Read the model definition and answer for the solid it produces. Units are mm, in the model's axes. A direction names the side the tool comes from. Coordinates: 2 decimals unless noted, no trailing zeros. Loops run counter-clockwise (first coordinate to the right, second up) from the corner with the lowest first, then second, coordinate; pieces in that order, holes last. Notation, with made-up numbers: (35, 68) - (40, 68) arc R25 cw to (40, 91) - close; hole circle Ø4 at (84.25, 56.5). An arc over 180 degrees is marked (long way). Use one line per item in the form item = value. Start each with the question number.
1) A cutting plane is placed at A-A (z = 0). Give the vertices of the cut face in (x, y) (3 decimals), and give its area (3 significant figures).
2) A cutting plane is placed at D-D (y = -2). Give the vertices of the cut face in (x, z) (3 decimals).
3) Consider line 1 (Z direction, x = 0, y = -32.75); line 2 (X direction, y = -1.5, z = 4.5) (3 decimals); line 3 (Y direction, x = -5.75, z = -13.5) (3 decimals). Determine where each line is inside the solid, lowest interval first.
4) This flat-tipped pin is pushed along its axis until it touches: P1, Ø5, axis at x = 0, z = 0, coming from the -Y side. Where does it stop, or does it pass through?
5) The mould has two halves that part along X. Classify faces 1 (the face through (0, -12.725, 5)), 2 (the face through (12.7, -9, 0)), 3 (the face through (-12.7, -9, 0)), 4 (the face through (9, 19.05, 0)): released by +X, released by -X, zero draft, split by the parting line, or undercut.
6) A cutting plane is placed at C-C (y = -16). Give the vertices of the cut face in (x, z), and give its area (3 significant figures).
7) Which of the six approach directions +Z, -Z, +X, -X, +Y, -Y give full straight-line access (tool end or side, diameter ignored) to faces 5 (the face through (6.375, 3, 0)), 6 (the face through (2.539, -25.247, -1.947))?
8) A cutting plane is placed at B-B (x = 0). Give the vertices of the cut face in (y, z) (3 decimals).
from build123d import *

# Parameters (mm, degrees)
F0_W      = 25.4
F0_H      = 38.1
F1_DEPTH  = 19.05
F2_T      = -6.325
F1_FACE_W = 25.4
F1_FACE_H = 38.1
F3_DEPTH  = 19.075
F5_D      = 6.4
F5_DEPTH  = 50


with BuildPart() as f1:
    # F0 (on Top) → F1 (new body, symmetric)
    with BuildSketch(Plane.XY):
        Rectangle(F0_W, F0_H)
    extrude(amount=F1_DEPTH, both=True)

    # F2
    f2_openings = [f1.faces().sort_by_distance(p)[0] for p in [
        (0, 19.05, 0),
        (0, 0, 19.05),
        (0, 0, -19.05),
    ]]
    offset(amount=F2_T, openings=f2_openings)

    # F1_face (on face) → F3 (join)
    with BuildSketch(Plane.XZ.offset(19.05)):
        Rectangle(F1_FACE_W, F1_FACE_H)
    extrude(amount=F3_DEPTH)

    # F5
    with Locations(Plane.XZ.offset(38.125)):
        with Locations((0, 0)):
            Hole(F5_D / 2, depth=F5_DEPTH)


solid = f1.part
Found:
q1.outline = (-12.7, -38.125) - (-3.2, -38.125) - (-3.2, -12.725) - (-6.375, -12.725) - (-6.375, 19.05) - (-12.7, 19.05) - close; (3.2, -38.125) - (12.7, -38.125) - (12.7, 19.05) - (6.375, 19.05) - (6.375, -12.725) - (3.2, -12.725) - close
q1.area = 885 mm^2
q2.outline = (-12.7, -19.05) - (-6.375, -19.05) - (-6.375, 19.05) - (-12.7, 19.05) - close; (6.375, -19.05) - (12.7, -19.05) - (12.7, 19.05) - (6.375, 19.05) - close
q3.line_1 = -19.05 to -3.2, 3.2 to 19.05
q3.line_2 = -12.7 to -6.375, 6.375 to 12.7
q3.line_3 = -38.125 to -12.725
q4.P1 = through
q5.face_1 = undercut
q5.face_2 = released by +X
q5.face_3 = released by -X
q5.face_4 = zero draft
q6.outline = (-12.7, -19.05) - (12.7, -19.05) - (12.7, 19.05) - (-12.7, 19.05) - close; hole circle Ø6.4 at (0, 0)
q6.area = 936 mm^2
q7.face_5 = +Z, -Z, +Y
q7.face_6 = +Y, -Y
q8.outline = (-38.125, -19.05) - (-12.725, -19.05) - (-12.725, -3.2) - (-38.125, -3.2) - close; (-38.125, 3.2) - (-12.725, 3.2) - (-12.725, 19.05) - (-38.125, 19.05) - close
